from build123d import *

# Parameters (mm, degrees)
F0_W        = 47.9449257255
F0_H        = 29.3166413903
F1_DEPTH    = 127
F3_R        = 12.4646622314
F4_DEPTH    = 127
F5_T1_DEPTH = 254
F6_T1_DEPTH = 194.7542070367
F7_T1_DEPTH = 194.7542070365


# Not quite as in the source:
# - a fillet or chamfer that OpenCascade refuses, or shapes differently, is made with other operations: its cross-section is extruded or revolved along the edge and cut away or added


with BuildPart() as f1:
    # F0 (on Front) → F1 (new body)
    with BuildSketch(Plane.XZ):
        with Locations((-23.9724628627, 14.6583206952)):
            Rectangle(F0_W, F0_H)
    extrude(amount=F1_DEPTH)

    # F3 (on face) → F4 (cut)
    with BuildSketch(Plane.XZ.offset(127)):
        with Locations((-23.5143899918, 14.3529390916)):
            Circle(F3_R)
    extrude(amount=-F4_DEPTH, mode=Mode.SUBTRACT)

    # F5: fillet of radius 25.4 on 2 edges, made by hand

    # F5_s2 → F5_t1 (cut)
    with BuildSketch(Plane.XZ.offset(-63.5)):
        with BuildLine():
            ThreePointArc((-47.9449257255, 3.9166413903), (-40.5054379676, 21.8771536325), (-22.5449257255, 29.3166413903))
            Line((-22.5449257255, 29.3166413903), (-47.9449257255, 29.3166413903))
            Line((-47.9449257255, 29.3166413903), (-47.9449257255, 3.9166413903))
        make_face()
        with BuildLine():
            ThreePointArc((0, 3.9166413903), (-7.4394877579, 21.8771536325), (-25.4, 29.3166413903))
            Line((-25.4, 29.3166413903), (0, 29.3166413903))
            Line((0, 29.3166413903), (0, 3.9166413903))
        make_face()
    extrude(amount=F5_T1_DEPTH, mode=Mode.SUBTRACT)

    # F6: fillet of radius 25.4 on 1 edges, made by hand

    # F6_s2 → F6_t1 (cut)
    with BuildSketch(Plane.XZ.offset(-33.8771035184)):
        with BuildLine():
            ThreePointArc((-13.5508414073, 0), (-6.4980869343, 0.9987980963), (0, 3.9166413903))
            Line((0, 3.9166413903), (0, 0))
            Line((0, 0), (-13.5508414073, 0))
        make_face()
    extrude(amount=F6_T1_DEPTH, mode=Mode.SUBTRACT)

    # F7: fillet of radius 25.4 on 1 edges, made by hand

    # F7_s2 → F7_t1 (cut)
    with BuildSketch(Plane.XZ.offset(-33.8771035183)):
        with BuildLine():
            ThreePointArc((-34.3940843182, 0), (-41.4468387912, 0.9987980963), (-47.9449257255, 3.9166413903))
            Line((-47.9449257255, 3.9166413903), (-47.9449257255, 0))
            Line((-47.9449257255, 0), (-34.3940843182, 0))
        make_face()
    extrude(amount=F7_T1_DEPTH, mode=Mode.SUBTRACT)


solid = f1.part
The model under review builds one solid part; all positions refer to its coordinate system, in mm. Round coordinates to 2 decimals unless told otherwise and drop trailing zeros. Loops run counter-clockwise (first coordinate to the right, second up) from the corner with the lowest first, then second, coordinate; pieces in that order, holes last. Notation, with made-up numbers: (51, 15.5) -> (86, 15.5) arc R23 ccw to (86, 39.5) -> close; hole circle Ø1 at (52, 32.5). An arc over 180 degrees is marked (long way). One line per question, with ' | ' between items. Start each with the question number.
Item 1: Draft analysis for pull direction X (two halves, no side actions). For faces 1 (the face through (-41.187, -62.611, 21.168)), 2 (the face through (-33.406, -64.389, 6.768)), 3 (the face through (-35, -127, 8)), state which applies: +X half, -X half, draft (parallel to the pull), parting line (faces both ways), or undercut.
Item 2: Wall thickness on line 1 along X through (y, z) = (-90.5, 7.5); line 2 along X through (y, z) = (-19, 16.5); line 3 along Z through (x, y) = (-31.5, -68.5): over which ranges is each line inside the solid? List them lowest first. Write a range as [from, to].
Item 3: Add section C-C, the plane y = -22.5. Write out the cut boundary in (x, z), then the cut area to 3 significant figures.
Item 4: Add section D-D, the plane x = -40. Write out the cut boundary in (y, z), then the cut area to 3 significant figures.
Item 5: For pin 1 (1 mm diameter, centred on x = -20, y = -26.5, fed in from +Z); pin 2 (1.5 mm diameter, centred on y = -107, z = 18.5, fed in from -X); pin 3 (1 mm diameter, centred on x = -28.5, y = -38, fed in from +Z), all flat-tipped, find the tip position at first contact; note any pin that passes through.
Item 6: Add section A-A, the plane x = -19.5. Write out the cut boundary in (y, z).
Item 7: Add section B-B, the plane z = 8.75. Write out the cut boundary in (x, y).
Return value:
1) face 1: -X half | face 2: undercut | face 3: draft
2) line 1: x = [-47.69, -33.93], [-13.1, -0.25] | line 2: x = [-44.61, -35.79], [-11.24, -3.34] | line 3: z = [0, 4.78], [23.92, 27.69]
3) outline: (-47.94, 3.92) arc R25.4 ccw to (-34.39, 0) -> (-13.55, 0) arc R25.4 ccw to (0, 3.92) arc R25.4 ccw to (-23.97, 29.28) arc R25.4 ccw to start; hole circle Ø24.93 at (-23.51, 14.35) | area: 606 mm2
4) outline: (-127, 0.63) -> (0, 0.63) -> (0, 22.37) -> (-127, 22.37) -> close | area: 2,760 mm2
5) pin 1: stops at z = 28.84 | pin 2: stops at x = -43.85 | pin 3: stops at z = 28.72
6) outline: (-127, 0) -> (0, 0) -> (0, 2.55) -> (-127, 2.55) -> close; (-127, 26.15) -> (0, 26.15) -> (0, 28.62) -> (-127, 28.62) -> close
7) outline: (-47.48, -127) -> (-34.65, -127) -> (-34.65, 0) -> (-47.48, 0) -> close; (-12.38, -127) -> (-0.46, -127) -> (-0.46, 0) -> (-12.38, 0) -> close
